For this review, use the dimensioned drawing (mm, ordinates from the lowest corner) and the shaded views. Coordinates: 2 decimals unless noted, no trailing zeros. Write each loop counter-clockwise with the first axis right and the second up, starting at its lowest first coordinate (ties: lowest second). Pieces come first, ordered by that corner, then holes. Notation, with made-up numbers: M -3,52 L 12,52 A21 cw 12,71 Z; hole C 29.5,-9 d1. An arc over 180 degrees is marked long. Return JSON: item names as keys, results as strings.
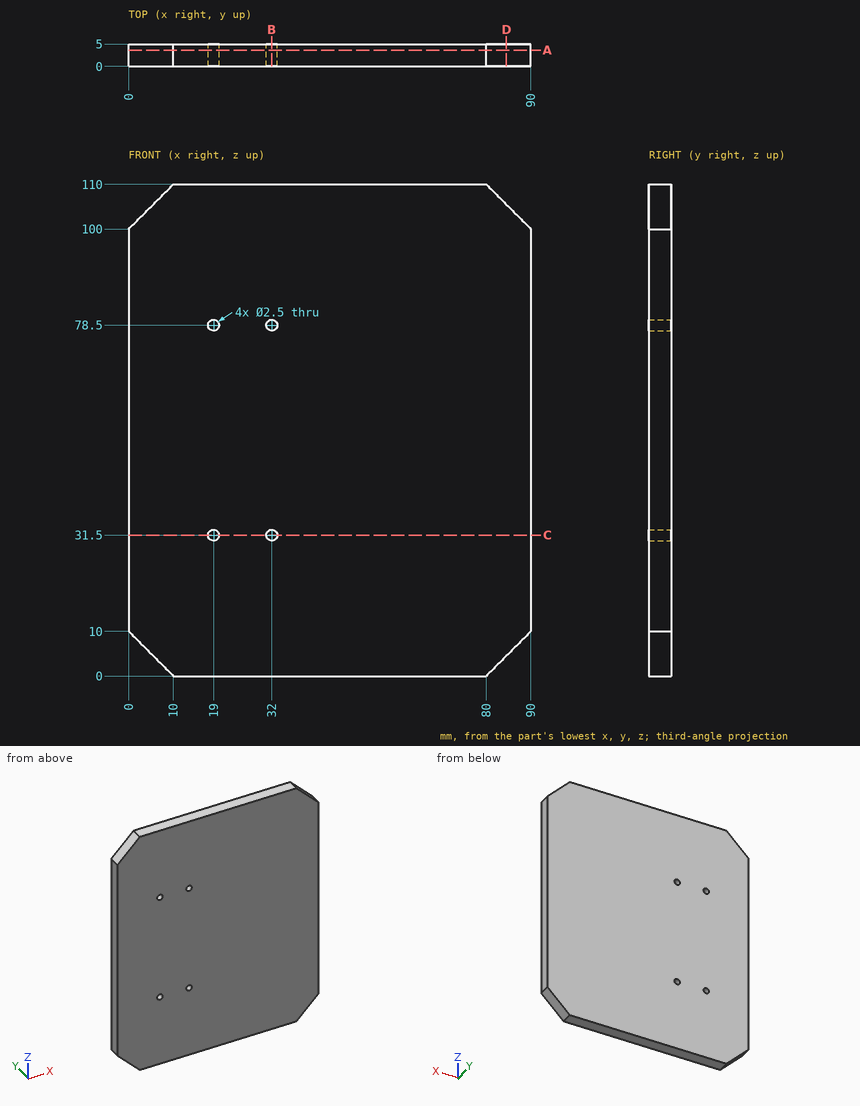
1. We need section B-B (x = 32). State the section outline as (y, z) points.
Checks:
{"outline": "M 0,0 L 5,0 L 5,30.25 L 0,30.25 Z; M 0,32.75 L 5,32.75 L 5,77.25 L 0,77.25 Z; M 0,79.75 L 5,79.75 L 5,110 L 0,110 Z"}
2. Wall thickness on L1, parallel to X at y = 1.2, z = 78.5; L2, parallel to Z at x = 19, y = 1.15; L3, parallel to X at y = 0.85, z = 78: over which ranges is each line inside the solid? List them lowest first. Write a range as from..to.
Checks:
{"L1": "0..17.75, 20.25..30.75, 33.25..90", "L2": "0..30.25, 32.75..77.25, 79.75..110", "L3": "0..17.85, 20.15..30.85, 33.15..90"}
3. We need section C-C (z = 31.5). State the section outline as (x, y) points, plus the area to 3 significant figures.
Checks:
{"outline": "M 0,0 L 17.75,0 L 17.75,5 L 0,5 Z; M 20.25,0 L 30.75,0 L 30.75,5 L 20.25,5 Z; M 33.25,0 L 90,0 L 90,5 L 33.25,5 Z", "area": "425 mm2"}
4. We need section D-D (x = 84.5). State the section outline as (y, z) points, plus the area to 3 significant figures.
Checks:
{"outline": "M 0,4.5 L 5,4.5 L 5,105.5 L 0,105.5 Z", "area": "505 mm2"}
5. We need section A-A (y = 3.65). State the section outline as (x, z) points.
Checks:
{"outline": "M 0,10 L 10,0 L 80,0 L 90,10 L 90,100 L 80,110 L 10,110 L 0,100 Z; hole C 19,31.5 d2.5; hole C 19,78.5 d2.5; hole C 32,31.5 d2.5; hole C 32,78.5 d2.5"}
